from build123d import *

# Parameters (mm, degrees)
SKETCH_2_R               = 2
CUT_EXTRUDE_1_DEPTH      = 10
CUT_EXTRUDE_1_DEPTH_BACK = 10


with BuildPart() as part:
    # Эскиз1 → Повернуть1 (revolve)
    with BuildSketch(Plane.XY, mode=Mode.PRIVATE) as revolve_1_sk:
        Polygon((-7.4, 9.1), (-7.4, 1), (-9, 1), (-9, 0), (-6.894121554, 0), (-6.894121554, -34.110992832), (-6, -35.9), (-6, 9.1), align=None)
    revolve(revolve_1_sk.sketch.rotate(Axis((0, 30.712290503, 0), (0, -1, 0)), 270), axis=Axis((0, 30.712290503, 0), (0, -1, 0)))  # turned: the seam where the file's is

    # Эскиз2 → Вырез-Вытянуть1 (cut, two sides)
    with BuildSketch(Plane.XY) as cut_extrude_1_sk:
        with Locations((0, -31.2)):
            Circle(SKETCH_2_R)
    extrude(amount=CUT_EXTRUDE_1_DEPTH, mode=Mode.SUBTRACT)
    extrude(cut_extrude_1_sk.sketch, amount=-CUT_EXTRUDE_1_DEPTH_BACK, mode=Mode.SUBTRACT)


solid = part.part
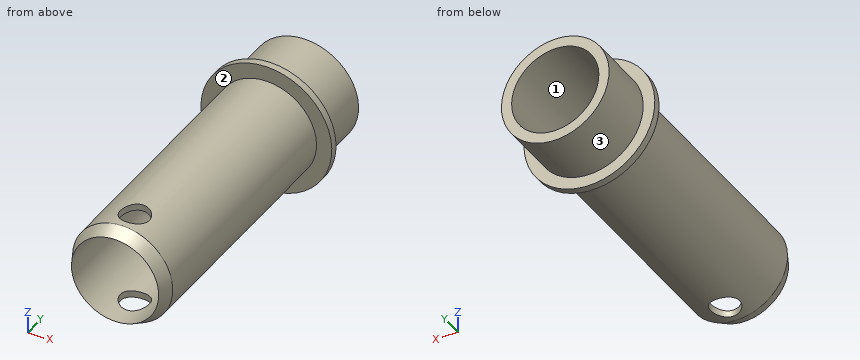
Can you work these out from the model? Positions are in its coordinate system, mm. Face numbers are marked on the shaded views. Give positions to 0.01 mm unless a question says otherwise; leave off trailing zeros. Order: outer loops, then holes, each group sorted by start corner. A loop starts at its lowest first (then second) coordinate and runs counter-clockwise, first axis right, second up. Notation, with made-up numbers: (8.25, -37.75) - (63.25, -37.75) arc R20 cw to (63.25, -16.75) - close; hole circle Ø11 at (76.25, 68.5). An arc over 180 degrees is marked (long way). Write each question's results on one line, items separated by ' | '.
1) Suppose I cut it at D-D, the plane y = 4. Write out the boundary of the cut face in (x, z).
Final values:
outline: circle Ø14.8 at (0, 0); hole circle Ø12 at (0, 0)
2) Please list where these lines run through material, in increasing order: line 1 along X through (y, z) = (-7.5, 0); line 2 along Z through (x, y) = (0.25, -18); line 3 along X through (y, z) = (4.5, 0.75). Write a range as [from, to].
Final values:
line 1: x = [-6.89, -6], [6, 6.89] | line 2: z = [-6.89, -5.99], [5.99, 6.89] | line 3: x = [-7.36, -5.95], [5.95, 7.36]
3) I'm going to push flat-ended pins straight in: pin 1 Ø10 at (y, z) = (-20, 3) entering from -X; pin 2 Ø4 at (y, z) = (4.5, 1) entering from -X; pin 3 Ø8 at (x, y) = (6.5, -18) entering from +Z. Where does each tip first touch, or does it pass through?
Final values:
pin 1: stops at x = -6.89 | pin 2: stops at x = -7.4 | pin 3: stops at z = 6.42
4) Suppose I cut it at C-C, the plane y = -31.2. Write out the boundary of the cut face in (x, z).
Final values:
outline: (-2, -6.6) - (-2, -5.66) arc R6 cw to (-2, 5.66) - (-2, 6.6) arc R6.89 ccw to start; (2, -6.6) arc R6.89 ccw to (2, 6.6) - (2, 5.66) arc R6 cw to (2, -5.66) - close
5) If we mould it in two halves opening along X, with no side actions, what happens to the marked faces 1, 2 and 3? For each: pulls with the +X half, pulls with the -X half, needs draft (parallel to the pull), parting line crosses it, or undercut.
Final values:
face 1: undercut | face 2: needs draft | face 3: parting line crosses it
6) Suppose I cut it at B-B, the plane x = 0. Write out the boundary of the cut face in (y, z).
Final values:
outline: (-35.9, -6) - (-34.11, -6.89) - (-33.2, -6.89) - (-33.2, -6) - close; (-35.9, 6) - (-33.2, 6) - (-33.2, 6.89) - (-34.11, 6.89) - close; (-29.2, -6.89) - (0, -6.89) - (0, -9) - (1, -9) - (1, -7.4) - (9.1, -7.4) - (9.1, -6) - (-29.2, -6) - close; (-29.2, 6) - (9.1, 6) - (9.1, 7.4) - (1, 7.4) - (1, 9) - (0, 9) - (0, 6.89) - (-29.2, 6.89) - close
7) Suppose I cut it at A-A, the plane z = 0. Write out the boundary of the cut face in (x, y).
Final values:
outline: (-9, 0) - (-6.89, 0) - (-6.89, -34.11) - (-6, -35.9) - (-6, 9.1) - (-7.4, 9.1) - (-7.4, 1) - (-9, 1) - close; (6, -35.9) - (6.89, -34.11) - (6.89, 0) - (9, 0) - (9, 1) - (7.4, 1) - (7.4, 9.1) - (6, 9.1) - close
